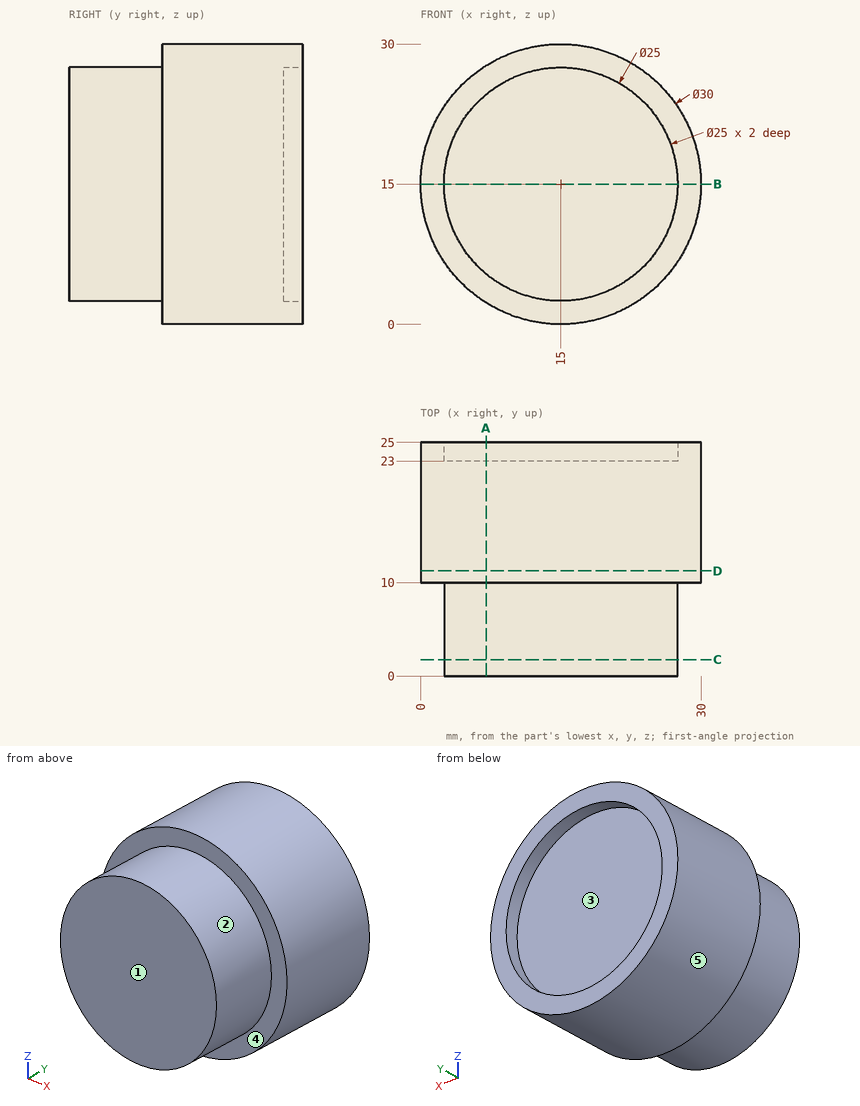
Geometry check sheet. Reference: drawing and pictorial views, mm from the part's lowest x, y, z. A direction names the side the tool comes from. Coordinates: 2 decimals unless noted, no trailing zeros. Order: outer loops, then holes, each group sorted by start corner. A loop starts at its lowest first (then second) coordinate and runs counter-clockwise, first axis right, second up.
Item 1: Section check B-B, the plane z = 15. Enter the section's corners in (x, y), then the cut area to 3 significant figures.
Filled in:
outline: (0, 10) - (2.5, 10) - (2.5, 0) - (27.5, 0) - (27.5, 10) - (30, 10) - (30, 25) - (27.5, 25) - (27.5, 23) - (2.5, 23) - (2.5, 25) - (0, 25) - close
area: 650 mm2
Item 2: Release check for a two-part mould opening along Z. For the marked faces 3, 4 and 5 record: +Z half, -Z half, draft (parallel to the pull), parting line (faces both ways), or undercut.
Filled in:
face 3: undercut
face 4: draft
face 5: parting line
Item 3: Section check C-C, the plane y = 1.75. Enter the section's corners in (x, z).
Filled in:
outline: circle Ø25 at (15, 15)
Item 4: Section check D-D, the plane y = 11.25. Enter the section's corners in (x, z).
Filled in:
outline: circle Ø30 at (15, 15)
Item 5: Section check A-A, the plane x = 7. Enter the section's corners in (y, z).
Filled in:
outline: (0, 5.4) - (10, 5.4) - (10, 2.31) - (25, 2.31) - (25, 5.4) - (23, 5.4) - (23, 24.6) - (25, 24.6) - (25, 27.69) - (10, 27.69) - (10, 24.6) - (0, 24.6) - close
Item 6: Material ranges on L1, parallel to X at y = 23.4, z = 15; L2, parallel to Z at x = 14.5, y = 2, recorded low to high.
Filled in:
L1: x = 0 to 2.5, 27.5 to 30
L2: z = 2.51 to 27.49
Item 7: Depth check by flat-ended pin: pin 1 (10 mm diameter, centred on x = 19.5, z = 16, fed in from +Y); pin 2 (1 mm diameter, centred on y = 8, z = 4, fed in from -X); pin 3 (3 mm diameter, centred on x = 22, y = 15.5, fed in from +Z). Enter the tip coordinate at first touch or a pass-through.
Filled in:
pin 1: stops at y = 23
pin 2: stops at x = 8.22
pin 3: stops at z = 28.96
Item 8: Access from +Z, -Z, +X, -X, +Y, -Y to the whole of each face (thin tool, end or side, straight path). Record for the marked faces 1 and 2.
Filled in:
face 1: +Z, -Z, +X, -X, -Y
face 2: -Y
